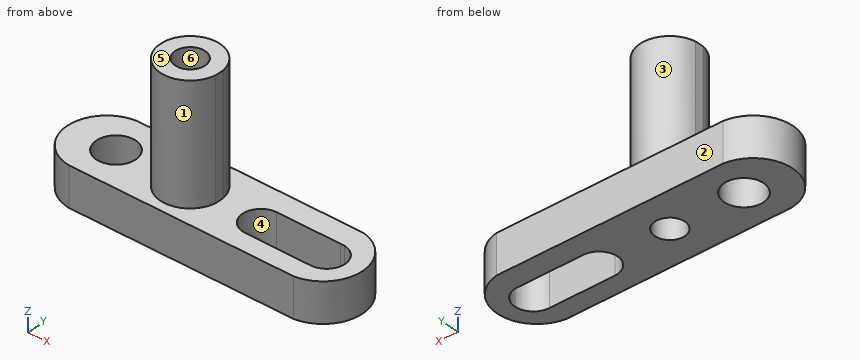
```python
from build123d import *

# Parameters (mm, degrees)
F1_DEPTH  = 25.4
F2_R      = 4.8404450777
F3_DEPTH  = 50.8
F5_DEPTH  = 25.4
F6_DEPTH  = 25.4
F7_R      = 6.3507472709
F8_DEPTH  = 25.4
F10_DEPTH = 38.1
F11_DEPTH = 25.4
F12_DEPTH = 25.4


# Not quite as in the source:
# - a feature names something its author has since deleted; it is built from what else it names


with BuildPart() as f1:
    # F0 (on Front) → F1 (new body)
    with BuildSketch(Plane.XZ):
        Polygon((-101.6, 0), (0, 0), (0, 12.7), (-49.7758105871, 12.7), (-49.7758105871, 50.8), (-68.8258105871, 50.8), (-68.8258105871, 12.7), (-101.6, 12.7), align=None)
    extrude(amount=F1_DEPTH)

    # F2 (on face) → F3 (cut)
    with BuildSketch(Plane.XY.offset(50.8)):
        with Locations((-59.3008105871, -12.7)):
            Circle(F2_R)
    extrude(amount=-F3_DEPTH, mode=Mode.SUBTRACT)

    # F4 (on face) → F5 (cut)
    with BuildSketch(Plane.XY.offset(12.7)):
        with BuildLine():
            ThreePointArc((-35.9137319028, -19.0677542063), (-31.7323936508, -17.3357871934), (-30.0004266379, -13.1544489413))
            ThreePointArc((-30.0004266379, -13.1544489413), (-31.7323936508, -8.9731106893), (-35.9137319028, -7.2411436764))
            ThreePointArc((-35.9137319028, -7.2411436764), (-41.8270371678, -13.1544489413), (-35.9137319028, -19.0677542063))
        make_face()
        with BuildLine():
            ThreePointArc((-35.9137319028, -7.2411436764), (-31.7323936508, -8.9731106893), (-30.0004266379, -13.1544489413))
            ThreePointArc((-30.0004266379, -13.1544489413), (-31.7323936508, -17.3357871934), (-35.9137319028, -19.0677542063))
            Line((-35.9137319028, -19.0677542063), (-14.5683543234, -19.1081041901))
            ThreePointArc((-14.5683543234, -19.1081041901), (-20.5006521622, -13.5013264467), (-15.2608531919, -7.2425229617))
            Line((-15.2608531919, -7.2425229617), (-35.9137319028, -7.2411436632))
        make_face()
        with BuildLine():
            Line((-13.852556963, -7.2426170145), (-15.2608531919, -7.2425229617))
            ThreePointArc((-15.2608531919, -7.2425229617), (-20.5006521622, -13.5013264467), (-14.5683543234, -19.1081041901))
            ThreePointArc((-14.5683543234, -19.1081041901), (-10.3512033015, -17.3683036228), (-8.603434015, -13.1544489413))
            ThreePointArc((-8.603434015, -13.1544489413), (-10.1050918857, -9.2015054667), (-13.852556963, -7.2426170145))
        make_face()
        with BuildLine():
            ThreePointArc((-13.852556963, -7.2426170145), (-14.5567022867, -7.2007830685), (-15.2608531919, -7.2425229617))
            Line((-15.2608531919, -7.2425229617), (-13.852556963, -7.2426170145))
        make_face()
        with BuildLine():
            ThreePointArc((-14.0938774664, 0), (-3.3585658021, -12.9691778388), (-14.712910818, -25.4))
            Line((-14.712910818, -25.4), (0, -25.4))
            Line((0, -25.4), (0, 0))
            Line((0, 0), (-14.0938774664, 0))
        make_face()
    extrude(amount=-F5_DEPTH, mode=Mode.SUBTRACT)

    # F4 (on face) → F6 (cut)
    with BuildSketch(Plane.XY.offset(12.7)):
        with BuildLine():
            ThreePointArc((-35.9137319028, -19.0677542063), (-31.7323936508, -17.3357871934), (-30.0004266379, -13.1544489413))
            ThreePointArc((-30.0004266379, -13.1544489413), (-31.7323936508, -8.9731106893), (-35.9137319028, -7.2411436764))
            ThreePointArc((-35.9137319028, -7.2411436764), (-41.8270371678, -13.1544489413), (-35.9137319028, -19.0677542063))
        make_face()
        with BuildLine():
            ThreePointArc((-35.9137319028, -7.2411436764), (-31.7323936508, -8.9731106893), (-30.0004266379, -13.1544489413))
            ThreePointArc((-30.0004266379, -13.1544489413), (-31.7323936508, -17.3357871934), (-35.9137319028, -19.0677542063))
            Line((-35.9137319028, -19.0677542063), (-14.5683543234, -19.1081041901))
            ThreePointArc((-14.5683543234, -19.1081041901), (-20.5006521622, -13.5013264467), (-15.2608531919, -7.2425229617))
            Line((-15.2608531919, -7.2425229617), (-35.9137319028, -7.2411436632))
        make_face()
        with BuildLine():
            Line((-13.852556963, -7.2426170145), (-15.2608531919, -7.2425229617))
            ThreePointArc((-15.2608531919, -7.2425229617), (-20.5006521622, -13.5013264467), (-14.5683543234, -19.1081041901))
            ThreePointArc((-14.5683543234, -19.1081041901), (-10.3512033015, -17.3683036228), (-8.603434015, -13.1544489413))
            ThreePointArc((-8.603434015, -13.1544489413), (-10.1050918857, -9.2015054667), (-13.852556963, -7.2426170145))
        make_face()
        with BuildLine():
            ThreePointArc((-13.852556963, -7.2426170145), (-14.5567022867, -7.2007830685), (-15.2608531919, -7.2425229617))
            Line((-15.2608531919, -7.2425229617), (-13.852556963, -7.2426170145))
        make_face()
    extrude(amount=-F6_DEPTH, mode=Mode.SUBTRACT)

    # F7 (on face) → F8 (cut)
    with BuildSketch(Plane.XY.offset(12.7)):
        with Locations((-83.2697451115, -12.8449322656)):
            Circle(F7_R)
        with BuildLine():
            ThreePointArc((-87.6296867998, -25.4), (-99.1786550293, -12.7), (-87.6296867998, 0))
            Line((-87.6296867998, 0), (-101.6, 0))
            Line((-101.6, 0), (-101.6, -25.4))
            Line((-101.6, -25.4), (-87.6296867998, -25.4))
        make_face()
    extrude(amount=-F8_DEPTH, mode=Mode.SUBTRACT)

    # F9 (on face) → F10 (cut)
    with BuildSketch(Plane.XY.offset(50.8)):
        with BuildLine():
            ThreePointArc((-68.8258105871, -11.3028298429), (-59.3008105871, -3.0730737279), (-49.7758105871, -11.3028298429))
            Line((-49.7758105871, -11.3028298429), (-49.7758105871, 0))
            Line((-49.7758105871, 0), (-68.8258105871, 0))
            Line((-68.8258105871, 0), (-68.8258105871, -11.3028298429))
        make_face()
        with BuildLine():
            Line((-49.7758105871, -25.4), (-49.7758105871, -14.0971701571))
            ThreePointArc((-49.7758105871, -14.0971701571), (-59.3008105871, -22.3269262721), (-68.8258105871, -14.0971701571))
            Line((-68.8258105871, -14.0971701571), (-68.8258105871, -25.4))
            Line((-68.8258105871, -25.4), (-49.7758105871, -25.4))
        make_face()
    extrude(amount=-F10_DEPTH, mode=Mode.SUBTRACT)


with BuildPart() as f11:
    # F7 (on face) → F11 (new body)
    with BuildSketch(Plane.XY.offset(12.7)):
        with Locations((-83.2697451115, -12.8449322656)):
            Circle(F7_R)
    extrude(amount=F11_DEPTH)

    # F12 (cut): a face of the model
    f12_faces = [f11.faces().sort_by_distance(p)[0] for p in [
        (-83.2697451115, -12.8449322656, 38.1),
    ]]
    extrude(f12_faces, amount=-F12_DEPTH, mode=Mode.SUBTRACT)


solid = f1.part
```
Check sheet for the modelled part. Datum: model origin and axes. Units: mm. Face numbers are marked on the shaded views. A direction names the side the tool comes from. Coordinates: 2 decimals unless noted, no trailing zeros. Loops run counter-clockwise (first coordinate to the right, second up) from the corner with the lowest first, then second, coordinate; pieces in that order, holes last. Notation, with made-up numbers: M 50.25,-5.5 L 82.25,-5.5 A25 ccw 82.25,24.5 Z; hole C 85,30 d2. An arc over 180 degrees is marked long. Answer as a JSON object with one key per item and string values.
1. Sectioned sample at A-A on z = 19. Record the cut outline in (x, y), and give its area (3 significant figures).
Outcome:
{"outline": "M -68.83,-14.1 A9.63 ccw -49.78,-14.1 L -49.78,-11.3 A9.63 ccw -68.83,-11.3 Z; hole C -59.3,-12.7 d9.68", "area": "217 mm²"}
2. Release check for a two-part mould opening along Y. For the marked faces 3, 4, 5 and 6 record: pulls with the +Y half, pulls with the -Y half, needs draft (parallel to the pull), parting line crosses it, or undercut.
Outcome:
{"face 3": "pulls with the +Y half", "face 4": "undercut", "face 5": "needs draft", "face 6": "undercut"}
3. Sectioned sample at D-D on z = 11.5. Record the cut outline in (x, y).
Outcome:
{"outline": "M -87.63,-25.4 L -14.71,-25.4 A12.83 ccw -14.09,0 L -87.63,0 A12.76 ccw Z; hole C -83.27,-12.84 d12.7; hole C -59.3,-12.7 d9.68; hole M -35.91,-19.07 L -14.57,-19.11 A5.95 ccw long -15.26,-7.24 L -35.91,-7.24 A5.91 ccw Z"}
4. Sectioned sample at C-C on y = -15. Record the cut outline in (x, z), and give its area (3 significant figures).
Outcome:
{"outline": "M -98.97,0 L -89.24,0 L -89.24,12.7 L -98.97,12.7 Z; M -77.3,0 L -63.56,0 L -63.56,50.8 L -68.65,50.8 L -68.65,12.7 L -77.3,12.7 Z; M -55.04,0 L -41.53,0 L -41.53,12.7 L -49.95,12.7 L -49.95,50.8 L -55.04,50.8 Z; M -8.9,0 L -3.57,0 L -3.57,12.7 L -8.9,12.7 Z", "area": "925 mm²"}
5. Scan lines: L1, parallel to X at y = -16.5, z = 11; L2, parallel to Z at x = -65, y = -3.25; L3, parallel to Y at x = -19, z = 3. Record each from-to range of solid material in increasing order. Write a range as from..to.
Outcome:
{"L1": "-98.6..-88.46, -78.08..-62.3, -56.3..-40.79, -9.63..-3.94", "L2": "0..12.7", "L3": "-25.4..-19.1, -7.24..0"}
6. Access from +Z, -Z, +X, -X, +Y, -Y to the whole of each face (thin tool, end or side, straight path). Record for the marked faces 1 and 2.
Outcome:
{"face 1": "+Z, -Y", "face 2": "+Z, -Z, +X, -X, +Y"}
7. Depth check by flat-ended pin: P1, Ø6, axis at y = -19, z = 24, coming from the -X side; P2, Ø2, axis at y = -13, z = 32, coming from the -X side; P3, Ø2, axis at y = -12, z = 35.5, coming from the +X side; P4, Ø10, axis at x = -83.27, y = -12.84, coming from the -Z side. Enter the tip coordinate at first touch or a pass-through.
Outcome:
{"P1": "x = -68.34", "P2": "x = -68.83", "P3": "x = -49.78", "P4": "through"}
8. Sectioned sample at B-B on x = -22. Record the cut outline in (y, z), and give its area (3 significant figures).
Outcome:
{"outline": "M -25.4,0 L -19.09,0 L -19.09,12.7 L -25.4,12.7 Z; M -7.24,0 L 0,0 L 0,12.7 L -7.24,12.7 Z", "area": "172 mm²"}
